Check sheet for the drawn part. Datum: minimum x, y, z corner. Units: mm. Coordinates: 2 decimals unless noted, no trailing zeros. Write each loop counter-clockwise with the first axis right and the second up, starting at its lowest first coordinate (ties: lowest second). Pieces come first, ordered by that corner, then holes. Notation, with made-up numbers: (84, 43) -> (90, 43) arc R10 cw to (90, 60) -> close; hole circle Ø6 at (-34, 86.5). An arc over 180 degrees is marked (long way). Write each question's results on one line, items separated by ' | '. Start each with the question number.
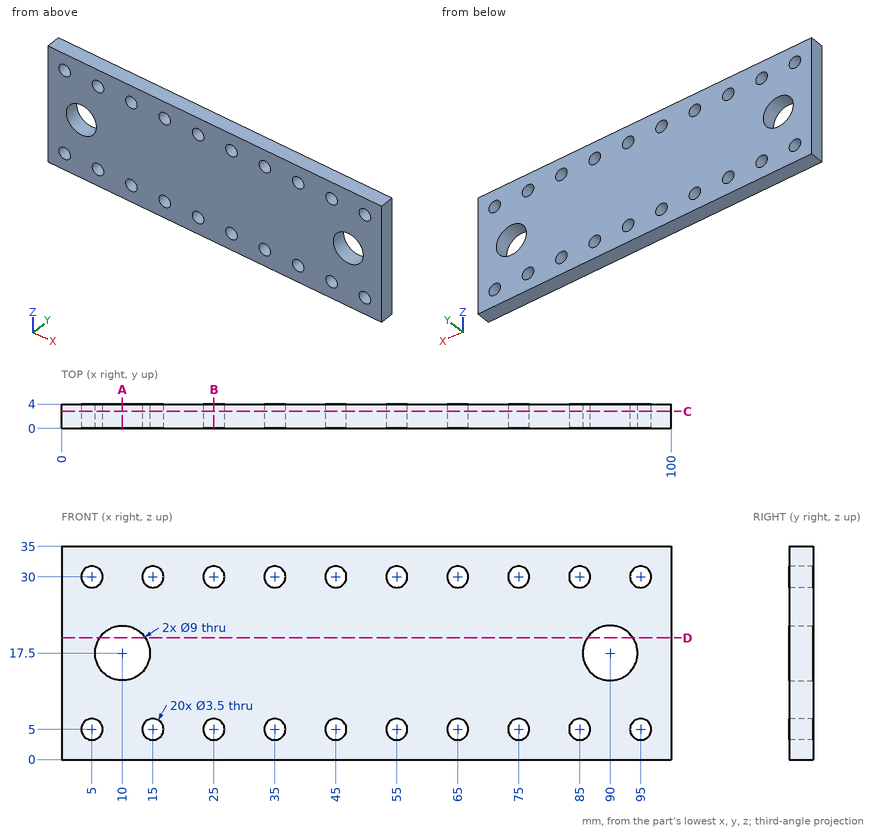
1. Sectioned sample at A-A on x = 10. Record the cut outline in (y, z), plus the area to 3 significant figures.
2. Material ranges on probe 1 along Z at (x, y) = (95, 2.7); probe 2 along X at (y, z) = (0.4, 18.5); probe 3 along Z at (x, y) = (86, 0.8), recorded low to high. Write a range as from..to.
3. Sectioned sample at D-D on z = 20. Record the cut outline in (x, y).
4. Sectioned sample at C-C on y = 2.8. State how many separate pieces and enclosed holes the cut face has, plus the area to 3 significant figures.
5. Sectioned sample at B-B on x = 25. Record the cut outline in (y, z).
Computed values:
1) outline: (0, 0) -> (4, 0) -> (4, 13) -> (0, 13) -> close; (0, 22) -> (4, 22) -> (4, 35) -> (0, 35) -> close | area: 104 mm^2
2) probe 1: z = 0..3.25, 6.75..28.25, 31.75..35 | probe 2: x = 0..5.61, 14.39..85.61, 94.39..100 | probe 3: z = 0..3.56, 6.44..15.44, 19.56..28.56, 31.44..35
3) outline: (0, 0) -> (6.26, 0) -> (6.26, 4) -> (0, 4) -> close; (13.74, 0) -> (86.26, 0) -> (86.26, 4) -> (13.74, 4) -> close; (93.74, 0) -> (100, 0) -> (100, 4) -> (93.74, 4) -> close
4) separate pieces: 1 | enclosed holes: 22 | area: 3,180 mm^2
5) outline: (0, 0) -> (4, 0) -> (4, 3.25) -> (0, 3.25) -> close; (0, 6.75) -> (4, 6.75) -> (4, 28.25) -> (0, 28.25) -> close; (0, 31.75) -> (4, 31.75) -> (4, 35) -> (0, 35) -> close
